Part model, mm, in its own coordinate system. Face numbers are marked on the shaded views. A direction names the side the tool comes from. Round coordinates to 2 decimals unless told otherwise and drop trailing zeros. Loops run counter-clockwise (first coordinate to the right, second up) from the corner with the lowest first, then second, coordinate; pieces in that order, holes last. Notation, with made-up numbers: (52, 39) - (92, 39) arc R19 cw to (92, 63) - close; hole circle Ø8 at (51.25, -2). An arc over 180 degrees is marked (long way). Put each result on its own line as item: value.
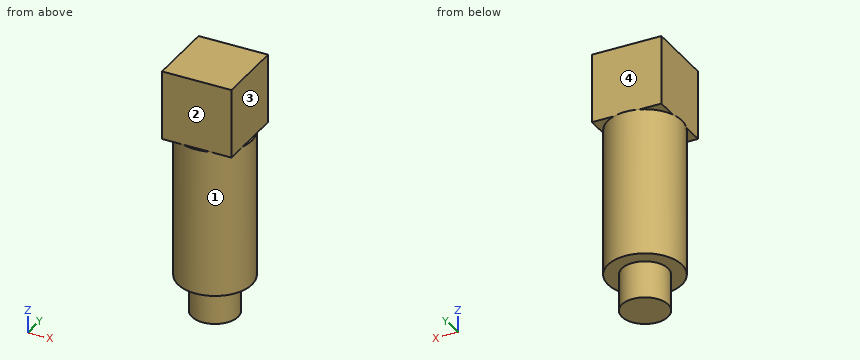
from build123d import *

# Parameters (mm, degrees)
SKETCH1_R           = 5
BOSS_EXTRUDE1_DEPTH = 8
SKETCH2_R           = 8
BOSS_EXTRUDE2_DEPTH = 32
SKETCH3_W           = 15
SKETCH3_H           = 15
BOSS_EXTRUDE3_DEPTH = 15


with BuildPart() as part:
    # Sketch1 → Boss-Extrude1 (new body)
    with BuildSketch(Plane.XY):
        Circle(SKETCH1_R)
    extrude(amount=BOSS_EXTRUDE1_DEPTH)

    # Sketch2 → Boss-Extrude2 (add)
    with BuildSketch(Plane.XY.offset(8)):
        Circle(SKETCH2_R)
    extrude(amount=BOSS_EXTRUDE2_DEPTH)

    # Sketch3 → Boss-Extrude3 (add)
    with BuildSketch(Plane.XY.offset(40)):
        Rectangle(SKETCH3_W, SKETCH3_H)
    extrude(amount=BOSS_EXTRUDE3_DEPTH)


solid = part.part
1. Pin check, flat tips, straight feed: P1, Ø1, axis at x = 6, z = 23, coming from the +Y side; P2, Ø4, axis at x = -4.5, y = -6.5, coming from the -Z side; P3, Ø5, axis at y = 5.5, z = 41, coming from the -X side. Stop position of each tip, or through.
A:
P1: stops at y = 5.81
P2: stops at z = 8
P3: stops at x = -7.5
2. Tool access for the marked faces 1, 2, 3 and 4: list every direction of +Z, -Z, +X, -X, +Y, -Y with a clear straight run to the whole face (end or side of a thin tool).
A:
face 1: -Z
face 2: +Z, +X, -X, -Y
face 3: +Z, +X, +Y, -Y
face 4: +Z, +X, -X, +Y
3. Probe line 1 along Z through (x, y) = (-6.5, -0.75); line 2 along X through (y, z) = (7, 42.5); line 3 along X through (y, z) = (3, 33.5). List the from-to ranges inside material, lowest first. Write a range as [from, to].
A:
line 1: z = [8, 55]
line 2: x = [-7.5, 7.5]
line 3: x = [-7.42, 7.42]
4. Band-saw the part on C-C (z = 4.5). List the corners of the cut face in (x, y), plus the area to 3 significant figures.
A:
outline: circle Ø10 at (0, 0)
area: 78.5 mm²
5. Band-saw the part on A-A (y = 0). List the corners of the cut face in (x, z).
A:
outline: (-8, 8) - (-5, 8) - (-5, 0) - (5, 0) - (5, 8) - (8, 8) - (8, 40) - (7.5, 40) - (7.5, 55) - (-7.5, 55) - (-7.5, 40) - (-8, 40) - close
6. Band-saw the part on D-D (y = 6.5). List the corners of the cut face in (x, z).
A:
outline: (-7.5, 40) - (-4.66, 40) - (-4.66, 8) - (4.66, 8) - (4.66, 40) - (7.5, 40) - (7.5, 55) - (-7.5, 55) - close
